from build123d import *

# Parameters (mm, degrees)
BOSS_EXTRUDE1_START = -40
SKETCH1_W           = 52
SKETCH1_H           = 3
BOSS_EXTRUDE1_DEPTH = 10
BOSS_EXTRUDE2_START = 20
SKETCH2_R           = 1.3
BOSS_EXTRUDE2_DEPTH = 6
BOSS_EXTRUDE3_START = 23.45
SKETCH3_R           = 2.3
BOSS_EXTRUDE3_DEPTH = 2.55
BOSS_EXTRUDE4_START = 20
SKETCH4_R           = 1.3
BOSS_EXTRUDE4_DEPTH = 6
BOSS_EXTRUDE5_START = 23.45
SKETCH5_R           = 2.3
BOSS_EXTRUDE5_DEPTH = 2.55


with BuildPart() as part:
    # Sketch1 → Boss-Extrude1 (new body)
    with BuildSketch(Plane.XY.offset(BOSS_EXTRUDE1_START)):
        with Locations((0, 23.25)):
            Rectangle(SKETCH1_W, SKETCH1_H)
    extrude(amount=BOSS_EXTRUDE1_DEPTH)


with BuildPart() as body_2:
    # Sketch2 → Boss-Extrude2 (new body)
    with BuildSketch(Plane(origin=(0, 0, 0), x_dir=(1, 0, 0), z_dir=(0, 1, 0)).offset(BOSS_EXTRUDE2_START)):
        with Locations(Location((-23.4, 35, 0), (0, 0, 270))):
            Circle(SKETCH2_R)
    extrude(amount=BOSS_EXTRUDE2_DEPTH)


with BuildPart() as part_1:
    add(part.part)

    # Combine1: cut body 2
    add(body_2.part, mode=Mode.SUBTRACT)


with BuildPart() as body_2_2:
    # Sketch3 → Boss-Extrude3 (new body)
    with BuildSketch(Plane(origin=(0, 0, 0), x_dir=(1, 0, 0), z_dir=(0, 1, 0)).offset(BOSS_EXTRUDE3_START)):
        with Locations(Location((-23.4, 35, 0), (0, 0, 270))):
            Circle(SKETCH3_R)
    extrude(amount=BOSS_EXTRUDE3_DEPTH)


with BuildPart() as part_2:
    add(part_1.part)

    # Combine2: cut body 2 2
    add(body_2_2.part, mode=Mode.SUBTRACT)


with BuildPart() as body_2_3:
    # Sketch4 → Boss-Extrude4 (new body)
    with BuildSketch(Plane(origin=(0, 0, 0), x_dir=(1, 0, 0), z_dir=(0, 1, 0)).offset(BOSS_EXTRUDE4_START)):
        with Locations(Location((23.4, 35, 0), (0, 0, 270))):
            Circle(SKETCH4_R)
    extrude(amount=BOSS_EXTRUDE4_DEPTH)


with BuildPart() as part_3:
    add(part_2.part)

    # Combine3: cut body 2 3
    add(body_2_3.part, mode=Mode.SUBTRACT)


with BuildPart() as body_2_4:
    # Sketch5 → Boss-Extrude5 (new body)
    with BuildSketch(Plane(origin=(0, 0, 0), x_dir=(1, 0, 0), z_dir=(0, 1, 0)).offset(BOSS_EXTRUDE5_START)):
        with Locations(Location((23.4, 35, 0), (0, 0, 270))):
            Circle(SKETCH5_R)
    extrude(amount=BOSS_EXTRUDE5_DEPTH)


with BuildPart() as part_4:
    add(part_3.part)

    # Combine4: cut body 2 4
    add(body_2_4.part, mode=Mode.SUBTRACT)


solid = part_4.part
Geometry check sheet. Reference: the model listing, model coordinates, mm. A direction names the side the tool comes from. Give positions to 0.01 mm unless a question says otherwise; leave off trailing zeros. Write each loop counter-clockwise with the first axis right and the second up, starting at its lowest first coordinate (ties: lowest second). Pieces come first, ordered by that corner, then holes.
1) Thickness scan on line 1 (X direction, y = 24.35, z = -35); line 2 (X direction, y = 22.8, z = -35); line 3 (Z direction, x = -23.4, y = 24.55). Record the ranges inside material, lowest first.
Values follow:
line 1: x = -26 to -25.7, -21.1 to 21.1, 25.7 to 26
line 2: x = -26 to -24.7, -22.1 to 22.1, 24.7 to 26
line 3: z = -40 to -37.3, -32.7 to -30
2) Cross-section at A-A (z = -35). Record the boundary of the cut face in (x, y), plus the area to 3 significant figures.
Values follow:
outline: (-26, 21.75) - (-24.7, 21.75) - (-24.7, 23.45) - (-25.7, 23.45) - (-25.7, 24.75) - (-26, 24.75) - close; (-22.1, 21.75) - (22.1, 21.75) - (22.1, 23.45) - (21.1, 23.45) - (21.1, 24.75) - (-21.1, 24.75) - (-21.1, 23.45) - (-22.1, 23.45) - close; (24.7, 21.75) - (26, 21.75) - (26, 24.75) - (25.7, 24.75) - (25.7, 23.45) - (24.7, 23.45) - close
area: 135 mm2
3) Cross-section at B-B (x = -23.4). Record the boundary of the cut face in (y, z).
Values follow:
outline: (21.75, -40) - (24.75, -40) - (24.75, -37.3) - (23.45, -37.3) - (23.45, -36.3) - (21.75, -36.3) - close; (21.75, -33.7) - (23.45, -33.7) - (23.45, -32.7) - (24.75, -32.7) - (24.75, -30) - (21.75, -30) - close
4) Set-up check for faces 5 (the face through (23.46, 22.59, -36.3)), 6 (the face through (-23, 23.45, -33)): record each of +Z, -Z, +X, -X, +Y, -Y from which the full face is reachable in a straight line by a thin tool's end or side.
Values follow:
face 5: +Y, -Y
face 6: +Y
5) Cross-section at C-C (y = 23). Record the boundary of the cut face in (x, z), plus the area to 3 significant figures.
Values follow:
outline: (-26, -40) - (26, -40) - (26, -30) - (-26, -30) - close; hole circle Ø2.6 at (-23.4, -35); hole circle Ø2.6 at (23.4, -35)
area: 509 mm2
6) Release check for a two-part mould opening along X. For faces 1 (the face through (26, 23, -35)), 2 (the face through (0, 23, -40)), 3 (the face through (22, 23.45, -34)), 4 (the face through (-26, 23, -35)) record: released by +X, released by -X, zero draft, split by the parting line, or undercut.
Values follow:
face 1: released by +X
face 2: zero draft
face 3: undercut
face 4: released by -X
7) Go/stop test with a flat-tipped pin: pin 1 Ø1.4 at (x, z) = (23, -36) entering from +Y. Record where the tip stops, or that it passes through.
Values follow:
pin 1: stops at y = 23.45
